The model under review builds one solid part; all positions refer to its coordinate system, in mm. Face numbers are marked on the shaded views. A direction names the side the tool comes from. Round coordinates to 2 decimals unless told otherwise and drop trailing zeros. Write each loop counter-clockwise with the first axis right and the second up, starting at its lowest first coordinate (ties: lowest second). Pieces come first, ordered by that corner, then holes.
Item 1: Draft analysis for pull direction X (two halves, no side actions). For the marked faces 1, 2, 3 and 4, state which applies: +X half, -X half, draft (parallel to the pull), parting line (faces both ways), or undercut.
Item 2: Add section B-B (x = 75). Give the boundary of the cut face in (y, z).
Item 3: Add section A-A (y = -5). Give the boundary of the cut face in (x, z).
Item 4: Clearance check with flat-ended pins moving along their axes: pin 1 Ø2 at (y, z) = (53, 4.5) entering from -X; pin 2 Ø5 at (x, z) = (78, 8.5) entering from +Y; pin 3 Ø3 at (x, y) = (74, 35.5) entering from -Z. State where each tip first meets the part, or that it passes through.
Item 5: Add section C-C (z = 6). State how many separate pieces and enclosed holes the cut face has, plus the area to 3 significant figures.
Item 6: Machinability: for the marked faces 5 and 6, which of the approach directions +Z, -Z, +X, -X, +Y, -Y give a long, thin tool a straight path to every point of the face, cutting with its end or side? Answer none if there is none.
Item 7: To check wall thickness, follow L1, parallel to X at y = -5, z = 4.5; L2, parallel to X at y = -3.5, z = 10.5; L3, parallel to Y at x = 59, z = 12.5. State the ranges of each line that lie inside material, in increasing order.
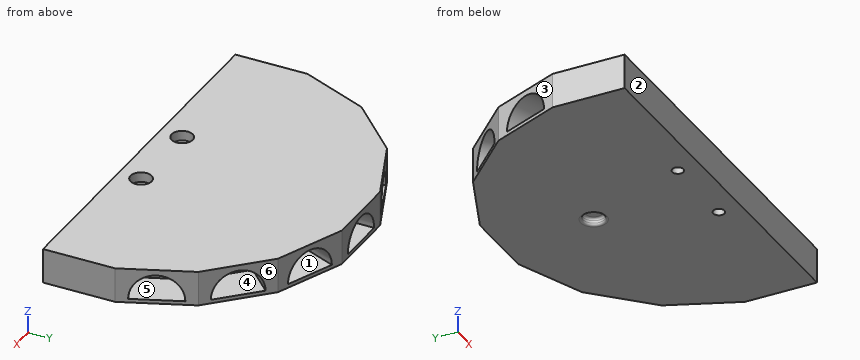
```python
from build123d import *

# Parameters (mm, degrees)
F0_W      = 150
F0_H      = 10
F0_R      = 2.25
F1_DEPTH  = 14
F5_DEPTH  = 15
F6_DEPTH  = 15
F7_DEPTH  = 15
F8_R      = 4.25
F9_DEPTH  = 4
F10_W     = 150
F10_H     = 14
F11_DEPTH = 4
F12_R     = 4.25
F13_DEPTH = 3
F14_R     = 1
F17_DEPTH = 15
F18_DEPTH = 15
F21_DEPTH = 15
F22_DEPTH = 15


with BuildPart() as f1:
    # F0 (on Top) → F1 (new body)
    with BuildSketch(Plane.XY):
        Polygon((0, 14.9184275535), (0, 0), (150, 0), (150, 14.9184275535), (138.5819298767, 42.4840873013), (117.4840873013, 63.5819298767), (89.9184275535, 75), (60.0815724465, 75), (32.5159126987, 63.5819298767), (11.4180701233, 42.4840873013), align=None)
        with Locations((75, -5)):
            Rectangle(F0_W, F0_H)
        with Locations((59, -5)):
            Circle(F0_R, mode=Mode.SUBTRACT)
        with Locations((91, -5)):
            Circle(F0_R, mode=Mode.SUBTRACT)
    extrude(amount=F1_DEPTH)

    # F4 (on face) → F5 (cut)
    with BuildSketch(Plane(origin=(90.533008589, 90.533008589, 0), x_dir=(-0.7071067812, 0.7071067812, 0), z_dir=(0.7071067812, 0.7071067812, 0))):
        with BuildLine():
            ThreePointArc((-42.783008589, 1.5), (-53.033008589, 11.75), (-63.283008589, 1.5))
            Line((-63.283008589, 1.5), (-42.783008589, 1.5))
        make_face()
    extrude(amount=-F5_DEPTH, mode=Mode.SUBTRACT)

    # F2 (on face) → F6 (cut)
    with BuildSketch(Plane(origin=(0, 75, 0), x_dir=(-1, 0, 0), z_dir=(0, 1, 0))):
        with BuildLine():
            ThreePointArc((-64.75, 1.5), (-75, 11.75), (-85.25, 1.5))
            Line((-85.25, 1.5), (-64.75, 1.5))
        make_face()
    extrude(amount=-F6_DEPTH, mode=Mode.SUBTRACT)

    # F3 (on face) → F7 (cut)
    with BuildSketch(Plane(origin=(-15.533008589, 15.533008589, 0), x_dir=(-0.7071067812, -0.7071067812, 0), z_dir=(-0.7071067812, 0.7071067812, 0))):
        with BuildLine():
            ThreePointArc((-42.783008589, 1.5), (-53.033008589, 11.75), (-63.283008589, 1.5))
            Line((-63.283008589, 1.5), (-42.783008589, 1.5))
        make_face()
    extrude(amount=-F7_DEPTH, mode=Mode.SUBTRACT)

    # F8 (on face) → F9 (cut)
    with BuildSketch(Plane.XY.offset(14)):
        with Locations((59, -5)):
            Circle(F8_R)
        with Locations((91, -5)):
            Circle(F8_R)
    extrude(amount=-F9_DEPTH, mode=Mode.SUBTRACT)

    # F10 (on face) → F11 (join)
    with BuildSketch(Plane.XZ.offset(10)):
        with Locations((75, 7)):
            Rectangle(F10_W, F10_H)
    extrude(amount=F11_DEPTH)

    # F12 (on face) → F13 (cut)
    with BuildSketch(Plane(origin=(0, 0, 0), x_dir=(1, 0, 0), z_dir=(0, 0, -1))):
        with Locations((75, -37)):
            Circle(F12_R)
    extrude(amount=-F13_DEPTH, mode=Mode.SUBTRACT)

    # F14
    f14_edges = [f1.edges().sort_by_distance(p)[0] for p in [
        (70.75, 37, 0),
        (70.75, 37, 3),
    ]]
    fillet(f14_edges, radius=F14_R)

    # F16 (on face) → F17 (cut)
    with BuildSketch(Plane(origin=(133.3074692328, 55.2177617219, 0), x_dir=(-0.3826834324, 0.9238795325, 0), z_dir=(0.9238795325, 0.3826834324, 0))):
        with BuildLine():
            ThreePointArc((-18.4512574274, 1.5), (-28.7012574274, 11.75), (-38.9512574274, 1.5))
            Line((-38.9512574274, 1.5), (-18.4512574274, 1.5))
        make_face()
    extrude(amount=-F17_DEPTH, mode=Mode.SUBTRACT)

    # F15 (on face) → F18 (cut)
    with BuildSketch(Plane(origin=(-5.2744606439, 2.1847531329, 0), x_dir=(-0.3826834324, -0.9238795325, 0), z_dir=(-0.9238795325, 0.3826834324, 0))):
        with BuildLine():
            ThreePointArc((-18.4512574274, 1.5), (-28.7012574274, 11.75), (-38.9512574274, 1.5))
            Line((-38.9512574274, 1.5), (-18.4512574274, 1.5))
        make_face()
    extrude(amount=-F18_DEPTH, mode=Mode.SUBTRACT)

    # F20 (on face) → F21 (cut)
    with BuildSketch(Plane(origin=(-17.7177617219, 42.7744606439, 0), x_dir=(-0.9238795325, -0.3826834324, 0), z_dir=(-0.3826834324, 0.9238795325, 0))):
        with BuildLine():
            ThreePointArc((-59.0409649383, 1.5), (-69.2909649383, 11.75), (-79.5409649383, 1.5))
            Line((-79.5409649383, 1.5), (-59.0409649383, 1.5))
        make_face()
    extrude(amount=-F21_DEPTH, mode=Mode.SUBTRACT)

    # F19 (on face) → F22 (cut)
    with BuildSketch(Plane(origin=(39.6847531329, 95.8074692328, 0), x_dir=(-0.9238795325, 0.3826834324, 0), z_dir=(0.3826834324, 0.9238795325, 0))):
        with BuildLine():
            ThreePointArc((-59.0409649383, 1.5), (-69.2909649383, 11.75), (-79.5409649383, 1.5))
            Line((-79.5409649383, 1.5), (-59.0409649383, 1.5))
        make_face()
    extrude(amount=-F22_DEPTH, mode=Mode.SUBTRACT)


solid = f1.part
```
Numbers:
1. face 1: undercut
1. face 2: draft
1. face 3: -X half
1. face 4: undercut
2. outline: (-14, 0) - (31.75, 0) arc R1 ccw to (32.75, 1) - (32.75, 2) arc R1 cw to (33.75, 3) - (40.25, 3) arc R1 cw to (41.25, 2) - (41.25, 1) arc R1 ccw to (42.25, 0) - (75, 0) - (75, 1.5) - (60, 1.5) - (60, 11.75) - (75, 11.75) - (75, 14) - (-14, 14) - close
3. outline: (0, 0) - (56.75, 0) - (56.75, 10) - (54.75, 10) - (54.75, 14) - (0, 14) - close; (61.25, 0) - (88.75, 0) - (88.75, 10) - (86.75, 10) - (86.75, 14) - (63.25, 14) - (63.25, 10) - (61.25, 10) - close; (93.25, 0) - (150, 0) - (150, 14) - (95.25, 14) - (95.25, 10) - (93.25, 10) - close
4. pin 1: stops at x = 34.76
4. pin 2: stops at y = 60
4. pin 3: stops at z = 3
5. separate pieces: 1
5. enclosed holes: 2
5. area: 9,090 mm2
6. face 5: none
6. face 6: +Z, -Z, +X, +Y
7. L1: x = 0 to 56.75, 61.25 to 88.75, 93.25 to 150
7. L2: x = 0 to 55.02, 62.98 to 87.02, 94.98 to 150
7. L3: y = -14 to -9.25, -0.75 to 74.55
